```python
from build123d import *

# Parameters (mm, degrees)
PAD002_DEPTH              = 2.5
CYLINDER005_R             = 2.8
CYLINDER005_DEPTH         = 15
CYLINDER004_R             = 1.5
CYLINDER004_DEPTH         = 8.5
FUSION002_PLACEMENT_ANGLE = 90
PAD001_DEPTH              = 2.5
CYLINDER003_R             = 2.8
CYLINDER003_DEPTH         = 15
CYLINDER002_R             = 1.5
CYLINDER002_DEPTH         = 8.5
FUSION001_PLACEMENT_ANGLE = 90
CYLINDER001_R             = 2
CYLINDER001_DEPTH         = 27.5
CYLINDER_R                = 2
CYLINDER_DEPTH            = 27.5
PAD_DEPTH                 = 10


with BuildPart() as body002:
    # Sketch002 → Pad002 (new body)
    with BuildSketch(Plane.XY):
        Polygon((0, -3.2), (2.771281, -1.6), (2.771281, 1.6), (0, 3.2), (-2.771281, 1.6), (-2.771281, -1.6), align=None)
    extrude(amount=PAD002_DEPTH)


with BuildPart() as cylinder005:
    # Cylinder005 → Cylinder005 (new body)
    with BuildSketch(Plane.XY.offset(5.5)):
        Circle(CYLINDER005_R)
    extrude(amount=CYLINDER005_DEPTH)


with BuildPart() as fusion002:
    # Cylinder004 → Cylinder004 (new body)
    with BuildSketch(Plane.XY):
        Circle(CYLINDER004_R)
    extrude(amount=CYLINDER004_DEPTH)

    # Fusion002: union Body002, Cylinder005
    add(body002.part)
    add(cylinder005.part)


with BuildPart() as fusion002_1:
    # Fusion002 placement: moved
    add(fusion002.part.moved(Location((93, 0, 0))).rotate(Axis((93, 0, 0), (-1, 0, 0)), FUSION002_PLACEMENT_ANGLE))


with BuildPart() as body001:
    # Sketch001 → Pad001 (new body)
    with BuildSketch(Plane.XY):
        Polygon((0, -3.2), (2.771281, -1.6), (2.771281, 1.6), (0, 3.2), (-2.771281, 1.6), (-2.771281, -1.6), align=None)
    extrude(amount=PAD001_DEPTH)


with BuildPart() as cylinder003:
    # Cylinder003 → Cylinder003 (new body)
    with BuildSketch(Plane.XY.offset(5.5)):
        Circle(CYLINDER003_R)
    extrude(amount=CYLINDER003_DEPTH)


with BuildPart() as fusion003:
    # Cylinder002 → Cylinder002 (new body)
    with BuildSketch(Plane.XY):
        Circle(CYLINDER002_R)
    extrude(amount=CYLINDER002_DEPTH)

    # Fusion001: union Body001, Cylinder003
    add(body001.part)
    add(cylinder003.part)


with BuildPart() as fusion003_1:
    # Fusion001 placement: moved
    add(fusion003.part.moved(Location((55, 0, 0))).rotate(Axis((55, 0, 0), (-1, 0, 0)), FUSION001_PLACEMENT_ANGLE))

    # Fusion003: union Fusion002
    add(fusion002_1.part)


with BuildPart() as cylinder001:
    # Cylinder001 → Cylinder001 (new body)
    with BuildSketch(Plane(origin=(130, 0, 0), x_dir=(1, 0, 0), z_dir=(0, 1, 0))):
        Circle(CYLINDER001_R)
    extrude(amount=CYLINDER001_DEPTH)


with BuildPart() as fusion:
    # Cylinder → Cylinder (new body)
    with BuildSketch(Plane(origin=(10, 0, 0), x_dir=(1, 0, 0), z_dir=(0, 1, 0))):
        Circle(CYLINDER_R)
    extrude(amount=CYLINDER_DEPTH)

    # Fusion: union Cylinder001
    add(cylinder001.part)


with BuildPart() as cut001:
    # Sketch (on Sketch) → Pad (new body, symmetric)
    with BuildSketch(Plane.XY):
        with BuildLine():
            Line((140, 0), (0, 0))
            Line((0, 0), (0, 27.499991))
            Line((0, 27.499991), (50, 27.499991))
            ThreePointArc((50, 27.499991), (52.460398, 16.914843), (59.337122, 8.5))
            Line((59.337122, 8.5), (88.662878, 8.5))
            ThreePointArc((88.662878, 8.5), (95.539604, 16.914847), (98, 27.5))
            Line((140, 27.5), (98, 27.5))
            Line((140, 27.5), (140, 0))
        make_face()
    extrude(amount=PAD_DEPTH, both=True)

    # Cut: cut Fusion
    add(fusion.part, mode=Mode.SUBTRACT)

    # Cut001: cut Fusion003
    add(fusion003_1.part, mode=Mode.SUBTRACT)


solid = cut001.part
```
Build history of the part. All positions in model axes, mm. A direction names the side the tool comes from. Round coordinates to 2 decimals unless told otherwise and drop trailing zeros. Write each loop counter-clockwise with the first axis right and the second up, starting at its lowest first coordinate (ties: lowest second). Pieces come first, ordered by that corner, then holes. Notation, with made-up numbers: (89.25, 61.25) - (107.25, 61.25) arc R13 cw to (107.25, 80.25) - close; hole circle Ø3 at (-2, 68). An arc over 180 degrees is marked (long way). Answer as CSV lines item,"result".
Q1. Drop flat-ended pins along their axis: pin 1 (5 mm diameter, centred on x = 93, z = 0, fed in from +Y); pin 2 (4.5 mm diameter, centred on x = 93, z = 0, fed in from -Y). Give the stop position or say it passes through.
Report:
pin 1,"stops at y = 5.5"
pin 2,"stops at y = 2.5"
Q2. Cut at C-C (z = -7.75). Write the cut outline in (x, y).
Report:
outline,"(0, 0) - (140, 0) - (140, 27.5) - (98, 27.5) arc R24 cw to (88.66, 8.5) - (59.34, 8.5) arc R24 cw to (50, 27.5) - (0, 27.5) - close"
Q3. Pull direction X, two halves, no side cores. Call faces 5 (the flat face through (25, 27.5, 0)), 6 (the cylindrical face through (56.43, 3.98, -0.45)), 7 (the flat face through (140, 14, 0)): +X half, -X half, draft (parallel to the pull), parting line (faces both ways), or undercut.
Report:
face 5,"draft"
face 6,"undercut"
face 7,"+X half"
Q4. Cut at D-D (y = 7). Write the cut outline in (x, z).
Report:
outline,"(0, -10) - (140, -10) - (140, 10) - (0, 10) - close; hole circle Ø4 at (10, 0); hole circle Ø5.6 at (55, 0); hole circle Ø5.6 at (93, 0); hole circle Ø4 at (130, 0)"
Q5. Cut at A-A (x = 130). Write the cut outline in (y, z), and give its area (3 significant figures).
Report:
outline,"(0, -10) - (27.5, -10) - (27.5, -2) - (0, -2) - close; (0, 2) - (27.5, 2) - (27.5, 10) - (0, 10) - close"
area,"440 mm^2"
Q6. Tool access for faces 1 (the cylindrical face through (96.45, 19.01, 0.14)), 2 (the flat face through (119, 27.5, 0)), 3 (the cylindrical face through (95.67, 10.07, -0.84)), 4 (the flat face through (90.229, 1, 0)): list every direction of +Z, -Z, +X, -X, +Y, -Y with a clear straight run to the whole face (end or side of a thin tool).
Report:
face 1,"+Z, -Z, +Y"
face 2,"+Z, -Z, +X, -X, +Y"
face 3,"+Y"
face 4,"-Y"
Q7. Cut at B-B (y = 23.25). Write the cut outline in (x, z), and give its area (3 significant figures).
Report:
outline,"(0, -10) - (50.38, -10) - (50.38, 10) - (0, 10) - close; (97.62, -10) - (140, -10) - (140, 10) - (97.62, 10) - close; hole circle Ø4 at (10, 0); hole circle Ø4 at (130, 0)"
area,"1,830 mm^2"
Q8. Drill centre lines: probe 1 along Z at (x, y) = (130, 21.5); probe 2 along X at (y, z) = (15, 9); probe 3 along Z at (x, y) = (55, 3.3). Where is each one in solid material? Low to high. Write a range as [from, to].
Report:
probe 1,"z = [-10, -2], [2, 10]"
probe 2,"x = [0, 53.51], [94.49, 140]"
probe 3,"z = [-10, -1.5], [1.5, 10]"
